Input: dimensioned drawing with shaded views. Units: mm. Origin: part minimum x, y, z. A direction names the side the tool comes from. Give positions to 0.01 mm unless a question says otherwise; leave off trailing zeros. Write each loop counter-clockwise with the first axis right and the second up, starting at its lowest first coordinate (ties: lowest second). Pieces come first, ordered by that corner, then holes. Notation, with made-up numbers: (70, -32.5) -> (119, -32.5) arc R17 cw to (119, -23.5) -> close; hole circle Ø9 at (-27.75, 21). An arc over 180 degrees is marked (long way). Answer in a Markdown table with one row per item. Add a question column.
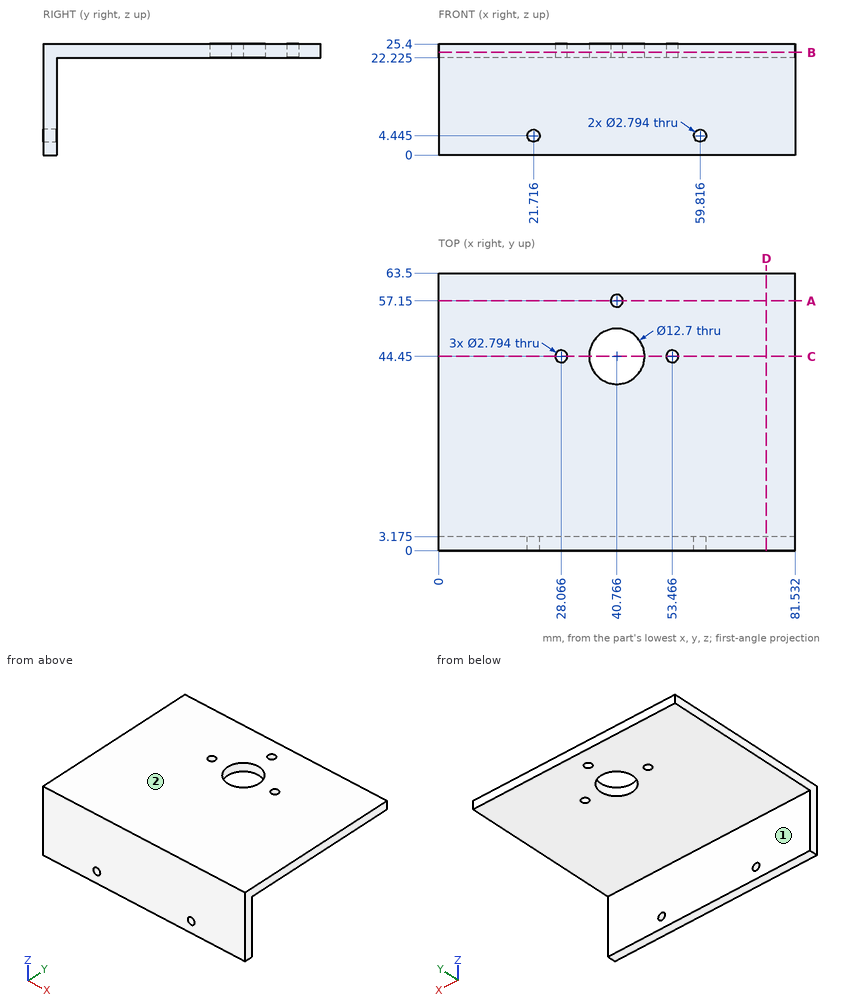
Q1. Section B-B on z = 23.5. Count the separate pieces of the cut face and the enclosed holes in it, and give its area (3 significant figures).
Q2. Section D-D on x = 75. Return loops of the section in (y, z) (1 decimal).
Q3. Line query: probe 1 along X at (y, z) = (45, 24.5); probe 2 along Y at (x, z) = (34, 18) (1 decimal); probe 3 along Z at (x, y) = (45, 10) (1 decimal). Output: solid intervals per line, ascending. Write a range as from..to.
Q4. Section A-A on y = 57.15. Return loops of the section in (x, z) (1 decimal), and give its area (3 significant figures).
Q5. Contact query for flat-ended pins moving along their axis: pin 1 Ø3.5 at (x, y) = (53.47, 44.45) entering from -Z (3 decimals); pin 2 Ø4.5 at (x, z) = (59.82, 4.44) entering from +Y (3 decimals). Output: stop coordinate, or through.
Q6. Section C-C on y = 44.45. Return loops of the section in (x, z) (1 decimal), and give its area (3 significant figures).
Q7. Access query for the marked faces 1 and 2. Directions: +Z, -Z, +X, -X, +Y, -Y. A direction counts if a zero-diameter tool reaches every point of the face in a straight line with its end or side. Return the directions, or none.
Checks:
| question | item | result |
|---|---|---|
| 1 | separate pieces | 1 |
| 1 | enclosed holes | 4 |
| 1 | area | 5,030 mm^2 |
| 2 | outline | (0, 0) -> (3.2, 0) -> (3.2, 22.2) -> (63.5, 22.2) -> (63.5, 25.4) -> (0, 25.4) -> close |
| 3 | probe 1 | 0..26.78, 29.35..34.44, 47.09..52.18, 54.75..81.53 |
| 3 | probe 2 | 0..3.2 |
| 3 | probe 3 | 22.2..25.4 |
| 4 | outline | (0, 22.2) -> (39.4, 22.2) -> (39.4, 25.4) -> (0, 25.4) -> close; (42.2, 22.2) -> (81.5, 22.2) -> (81.5, 25.4) -> (42.2, 25.4) -> close |
| 4 | area | 250 mm^2 |
| 5 | pin 1 | z = 22.225 |
| 5 | pin 2 | y = 3.175 |
| 6 | outline | (0, 22.2) -> (26.7, 22.2) -> (26.7, 25.4) -> (0, 25.4) -> close; (29.5, 22.2) -> (34.4, 22.2) -> (34.4, 25.4) -> (29.5, 25.4) -> close; (47.1, 22.2) -> (52.1, 22.2) -> (52.1, 25.4) -> (47.1, 25.4) -> close; (54.9, 22.2) -> (81.5, 22.2) -> (81.5, 25.4) -> (54.9, 25.4) -> close |
| 6 | area | 201 mm^2 |
| 7 | face 1 | -Z, +X, -X, +Y |
| 7 | face 2 | +Z, +X, -X, +Y, -Y |
